Check sheet for the modelled part. Datum: model origin and axes. Units: mm. Round coordinates to 2 decimals unless told otherwise and drop trailing zeros. Write each loop counter-clockwise with the first axis right and the second up, starting at its lowest first coordinate (ties: lowest second). Pieces come first, ordered by that corner, then holes.
Item 1: Section check A-A, the plane x = 102. Record the cut outline in (y, z) (3 decimals).
Item 2: Section check B-B, the plane y = -1.75. State how many separate pieces and enclosed holes the cut face has, plus the area to 3 significant figures.
Item 3: Release check for a two-part mould opening along X. For faces 1 (the flat face through (-82.783, -2, 0)), 2 (the flat face through (17, -2, -24.973)), 3 (the cylindrical face through (65.4, -1.57, 18.59)) record: pulls with the +X half, pulls with the -X half, needs draft (parallel to the pull), parting line crosses it, or undercut.
Item 4: Material ranges on line 1 along Z through (x, y) = (38, -0.9); line 2 along Z through (x, y) = (26.5, -0.9), recorded low to high.
from build123d import *

# Parameters (mm, degrees)
F0_W     = 203.2
F0_H     = 50.8
F0_R     = 2.3114
F1_DEPTH = 3.175


with BuildPart() as f1:
    # F0 (on Front) → F1 (new body)
    with BuildSketch(Plane.XZ):
        with Locations((18.816542, 0.427479)):
            Rectangle(F0_W, F0_H)
        with Locations((-76.433461, -18.622521)):
            Circle(F0_R, mode=Mode.SUBTRACT)
        with Locations((-63.733461, -18.622521)):
            Circle(F0_R, mode=Mode.SUBTRACT)
        with Locations((-51.033461, -18.622521)):
            Circle(F0_R, mode=Mode.SUBTRACT)
        with Locations((-38.333461, -18.622521)):
            Circle(F0_R, mode=Mode.SUBTRACT)
        with Locations((-25.633461, -18.622521)):
            Circle(F0_R, mode=Mode.SUBTRACT)
        with Locations((-12.933461, -18.622521)):
            Circle(F0_R, mode=Mode.SUBTRACT)
        with Locations((-0.233461, -18.622521)):
            Circle(F0_R, mode=Mode.SUBTRACT)
        with Locations((12.466539, -18.622521)):
            Circle(F0_R, mode=Mode.SUBTRACT)
        with Locations((-76.43346, -5.922521)):
            Circle(F0_R, mode=Mode.SUBTRACT)
        with Locations((-63.73346, -5.922521)):
            Circle(F0_R, mode=Mode.SUBTRACT)
        with Locations((-51.03346, -5.922521)):
            Circle(F0_R, mode=Mode.SUBTRACT)
        with Locations((-38.33346, -5.922521)):
            Circle(F0_R, mode=Mode.SUBTRACT)
        with Locations((-25.63346, -5.922521)):
            Circle(F0_R, mode=Mode.SUBTRACT)
        with Locations((-12.93346, -5.922521)):
            Circle(F0_R, mode=Mode.SUBTRACT)
        with Locations((-0.23346, -5.922521)):
            Circle(F0_R, mode=Mode.SUBTRACT)
        with Locations((12.46654, -5.922521)):
            Circle(F0_R, mode=Mode.SUBTRACT)
        with Locations((25.166539, -18.622521)):
            Circle(F0_R, mode=Mode.SUBTRACT)
        with Locations((37.866539, -18.622521)):
            Circle(F0_R, mode=Mode.SUBTRACT)
        with Locations((50.566539, -18.622521)):
            Circle(F0_R, mode=Mode.SUBTRACT)
        with Locations((63.266539, -18.622521)):
            Circle(F0_R, mode=Mode.SUBTRACT)
        with Locations((75.966539, -18.622521)):
            Circle(F0_R, mode=Mode.SUBTRACT)
        with Locations((88.666539, -18.622521)):
            Circle(F0_R, mode=Mode.SUBTRACT)
        with Locations((101.366539, -18.622521)):
            Circle(F0_R, mode=Mode.SUBTRACT)
        with Locations((114.066539, -18.622521)):
            Circle(F0_R, mode=Mode.SUBTRACT)
        with Locations((25.16654, -5.922521)):
            Circle(F0_R, mode=Mode.SUBTRACT)
        with Locations((37.86654, -5.922521)):
            Circle(F0_R, mode=Mode.SUBTRACT)
        with Locations((50.56654, -5.922521)):
            Circle(F0_R, mode=Mode.SUBTRACT)
        with Locations((63.26654, -5.922521)):
            Circle(F0_R, mode=Mode.SUBTRACT)
        with Locations((75.96654, -5.922521)):
            Circle(F0_R, mode=Mode.SUBTRACT)
        with Locations((88.66654, -5.922521)):
            Circle(F0_R, mode=Mode.SUBTRACT)
        with Locations((101.36654, -5.922521)):
            Circle(F0_R, mode=Mode.SUBTRACT)
        with Locations((114.06654, -5.922521)):
            Circle(F0_R, mode=Mode.SUBTRACT)
        with Locations((-76.433459, 6.777479)):
            Circle(F0_R, mode=Mode.SUBTRACT)
        with Locations((-63.733459, 6.777479)):
            Circle(F0_R, mode=Mode.SUBTRACT)
        with Locations((-51.033459, 6.777479)):
            Circle(F0_R, mode=Mode.SUBTRACT)
        with Locations((-38.333459, 6.777479)):
            Circle(F0_R, mode=Mode.SUBTRACT)
        with Locations((-25.633459, 6.777479)):
            Circle(F0_R, mode=Mode.SUBTRACT)
        with Locations((-12.933459, 6.777479)):
            Circle(F0_R, mode=Mode.SUBTRACT)
        with Locations((-0.233459, 6.777479)):
            Circle(F0_R, mode=Mode.SUBTRACT)
        with Locations((12.466541, 6.777479)):
            Circle(F0_R, mode=Mode.SUBTRACT)
        with Locations((-76.433458, 19.477479)):
            Circle(F0_R, mode=Mode.SUBTRACT)
        with Locations((-63.733458, 19.477479)):
            Circle(F0_R, mode=Mode.SUBTRACT)
        with Locations((-51.033458, 19.477479)):
            Circle(F0_R, mode=Mode.SUBTRACT)
        with Locations((-38.333458, 19.477479)):
            Circle(F0_R, mode=Mode.SUBTRACT)
        with Locations((-25.633458, 19.477479)):
            Circle(F0_R, mode=Mode.SUBTRACT)
        with Locations((-12.933458, 19.477479)):
            Circle(F0_R, mode=Mode.SUBTRACT)
        with Locations((-0.233458, 19.477479)):
            Circle(F0_R, mode=Mode.SUBTRACT)
        with Locations((12.466542, 19.477479)):
            Circle(F0_R, mode=Mode.SUBTRACT)
        with Locations((25.166541, 6.777479)):
            Circle(F0_R, mode=Mode.SUBTRACT)
        with Locations((37.866541, 6.777479)):
            Circle(F0_R, mode=Mode.SUBTRACT)
        with Locations((50.566541, 6.777479)):
            Circle(F0_R, mode=Mode.SUBTRACT)
        with Locations((63.266541, 6.777479)):
            Circle(F0_R, mode=Mode.SUBTRACT)
        with Locations((75.966541, 6.777479)):
            Circle(F0_R, mode=Mode.SUBTRACT)
        with Locations((88.666541, 6.777479)):
            Circle(F0_R, mode=Mode.SUBTRACT)
        with Locations((101.366541, 6.777479)):
            Circle(F0_R, mode=Mode.SUBTRACT)
        with Locations((114.066541, 6.777479)):
            Circle(F0_R, mode=Mode.SUBTRACT)
        with Locations((25.166542, 19.477479)):
            Circle(F0_R, mode=Mode.SUBTRACT)
        with Locations((37.866542, 19.477479)):
            Circle(F0_R, mode=Mode.SUBTRACT)
        with Locations((50.566542, 19.477479)):
            Circle(F0_R, mode=Mode.SUBTRACT)
        with Locations((63.266542, 19.477479)):
            Circle(F0_R, mode=Mode.SUBTRACT)
        with Locations((75.966542, 19.477479)):
            Circle(F0_R, mode=Mode.SUBTRACT)
        with Locations((88.666542, 19.477479)):
            Circle(F0_R, mode=Mode.SUBTRACT)
        with Locations((101.366542, 19.477479)):
            Circle(F0_R, mode=Mode.SUBTRACT)
        with Locations((114.066542, 19.477479)):
            Circle(F0_R, mode=Mode.SUBTRACT)
    extrude(amount=F1_DEPTH)


solid = f1.part
Values found:
1. outline: (-3.175, -24.973) - (0, -24.973) - (0, -20.845) - (-3.175, -20.845) - close; (-3.175, -16.4) - (0, -16.4) - (0, -8.145) - (-3.175, -8.145) - close; (-3.175, -3.7) - (0, -3.7) - (0, 4.555) - (-3.175, 4.555) - close; (-3.175, 9) - (0, 9) - (0, 17.255) - (-3.175, 17.255) - close; (-3.175, 21.7) - (0, 21.7) - (0, 25.827) - (-3.175, 25.827) - close
2. separate pieces: 1
2. enclosed holes: 64
2. area: 9,250 mm2
3. face 1: pulls with the -X half
3. face 2: needs draft
3. face 3: undercut
4. line 1: z = -24.97 to -20.93, -16.31 to -8.23, -3.61 to 4.47, 9.09 to 17.17, 21.79 to 25.83
4. line 2: z = -24.97 to -20.51, -16.73 to -7.81, -4.03 to 4.89, 8.67 to 17.59, 21.37 to 25.83
